Here's how the part is built. I have some questions about the finished solid (model axes, mm). A direction names the side the tool comes from. Give positions to 0.01 mm unless a question says otherwise; leave off trailing zeros. Loops run counter-clockwise (first coordinate to the right, second up) from the corner with the lowest first, then second, coordinate; pieces in that order, holes last. Notation, with made-up numbers: (44, -17.75) - (68, -17.75) arc R7 cw to (68, -7.75) - close; hole circle Ø9 at (56.25, -39.5). An arc over 180 degrees is marked (long way). Use a Markdown table: item, result.
from build123d import *

# Parameters (mm, degrees)
SKETCH2_R           = 4.60375
BOSS_EXTRUDE1_DEPTH = 127
SKETCH3_W           = 76.2
SKETCH3_H           = 31.474420728
CUT_EXTRUDE1_DEPTH  = 254
FILLET1_R           = 2.54
FILLET2_R           = 2.54
FILLET3_R           = 2.54
FILLET4_R           = 2.54
SKETCH4_R           = 1
SKETCH4_W           = 3.81
SKETCH4_H           = 10.16
CUT_EXTRUDE2_DEPTH  = 254


with BuildPart() as part:
    # Sketch2 → Boss-Extrude1 (new body)
    with BuildSketch(Plane.XY):
        with BuildLine():
            Line((-25.661451909, -36.676833639), (-25.661451909, -43.661833639))
            ThreePointArc((-25.661451909, -43.661833639), (-24.917503133, -45.457884863), (-23.121451909, -46.201833639))
            Line((-23.121451909, -46.201833639), (79.748548091, -46.201833639))
            ThreePointArc((79.748548091, -46.201833639), (81.544599316, -45.457884863), (82.288548091, -43.661833639))
            Line((82.288548091, -43.661833639), (82.288548091, -36.676833639))
            ThreePointArc((82.288548091, -36.676833639), (91.813548091, -27.151833639), (101.338548091, -36.676833639))
            Line((101.338548091, -36.676833639), (101.338548091, -46.201833639))
            Line((101.338548091, -46.201833639), (101.338548091, -46.836833639))
            ThreePointArc((101.338548091, -46.836833639), (98.92071457, -52.674000118), (93.083548091, -55.091833639))
            Line((93.083548091, -55.091833639), (-36.456451909, -55.091833639))
            ThreePointArc((-36.456451909, -55.091833639), (-42.293618387, -52.674000118), (-44.711451909, -46.836833639))
            Line((-44.711451909, -46.836833639), (-44.711451909, -46.201833639))
            Line((-44.711451909, -46.201833639), (-44.711451909, -36.676833639))
            ThreePointArc((-44.711451909, -36.676833639), (-35.186451909, -27.151833639), (-25.661451909, -36.676833639))
        make_face()
        with Locations((-35.186451909, -36.676833639)):
            Circle(SKETCH2_R, mode=Mode.SUBTRACT)
        with Locations((91.813548091, -36.676833639)):
            Circle(SKETCH2_R, mode=Mode.SUBTRACT)
    extrude(amount=-BOSS_EXTRUDE1_DEPTH)

    # Sketch3 → Cut-Extrude1 (cut)
    with BuildSketch(Plane(origin=(101.338548091, 0, 0), x_dir=(0, 0, -1), z_dir=(1, 0, 0))):
        with Locations((63.5, -30.464623275)):
            Rectangle(SKETCH3_W, SKETCH3_H)
    extrude(amount=-CUT_EXTRUDE1_DEPTH, mode=Mode.SUBTRACT)

    # Fillet1
    fillet1_edges = [part.edges().sort_by_distance(p)[0] for p in [
        (-33.916451909, -46.201833639, -25.4),
    ]]
    fillet(fillet1_edges, radius=FILLET1_R)

    # Fillet2
    fillet2_edges = [part.edges().sort_by_distance(p)[0] for p in [
        (-33.916451909, -46.201833639, -101.6),
    ]]
    fillet(fillet2_edges, radius=FILLET2_R)

    # Fillet3
    fillet3_edges = [part.edges().sort_by_distance(p)[0] for p in [
        (90.543548091, -46.201833639, -101.6),
    ]]
    fillet(fillet3_edges, radius=FILLET3_R)

    # Fillet4
    fillet4_edges = [part.edges().sort_by_distance(p)[0] for p in [
        (90.543548091, -46.201833639, -25.4),
    ]]
    fillet(fillet4_edges, radius=FILLET4_R)

    # Sketch4 → Cut-Extrude2 (cut)
    with BuildSketch(Plane(origin=(0, -46.201833639, 0), x_dir=(1, 0, 0), z_dir=(0, 1, 0))):
        with Locations(Location((-4.185751909, 106.86, 0), (0, 0, 270))):
            Circle(SKETCH4_R)
        with Locations(Location((60.814248091, 106.86, 0), (0, 0, 270))):
            Circle(SKETCH4_R)
        with Locations(Location((-4.185751909, 22.86, 0), (0, 0, 270))):
            Circle(SKETCH4_R)
        with Locations(Location((60.814248091, 22.86, 0), (0, 0, 270))):
            Circle(SKETCH4_R)
        with Locations((-16.250739794, 64.844309946)):
            Rectangle(SKETCH4_W, SKETCH4_H)
    extrude(amount=-CUT_EXTRUDE2_DEPTH, mode=Mode.SUBTRACT)


solid = part.part
(1) We'd pull the mould along Z, two halves only. Please class faces 1 (the face through (101.339, -42, -20)), 2 (the face through (-35.1, -31.9, -101.6)), 3 (the face through (29, -47, 0)): pulls with the +Z half, pulls with the -Z half, needs draft (parallel to the pull), parting line crosses it, or undercut.
A:
| item | result |
|---|---|
| face 1 | needs draft |
| face 2 | undercut |
| face 3 | pulls with the +Z half |
(2) If I drill on line 1 (X direction, y = -48.5, z = -22.86); line 2 (Y direction, x = 92, z = -6); line 3 (X direction, y = -52.75, z = -106.86), over which ranges is the centre line in solid material (lowest first)?
A:
| item | result |
|---|---|
| line 1 | -44.54 to -5.19, -3.19 to 59.81, 61.81 to 101.17 |
| line 2 | -55.09 to -41.28, -32.08 to -27.15 |
| line 3 | -42.22 to -5.19, -3.19 to 59.81, 61.81 to 98.84 |
(3) Suppose I cut it at A-A on z = -7.5. Count the separate pieces of the cut face and the enclosed holes in it, plus the area to 3 significant figures.
A:
| item | result |
|---|---|
| separate pieces | 1 |
| enclosed holes | 2 |
| area | 1,790 mm2 |
(4) Will this pin go through, and if not, where does the flat tip stop? pin 1 (10 mm diameter, centred on x = 60, z = -81, fed in from +Y).
A:
| item | result |
|---|---|
| pin 1 | y = -46.2 |
(5) Suppose I cut it at B-B on y = -50.75. Write out the boundary of the cut face in (x, z).
A:
| item | result |
|---|---|
| outline | (-43.73, -127) - (100.35, -127) - (100.35, 0) - (-43.73, 0) - close; hole (-18.16, -69.92) - (-14.35, -69.92) - (-14.35, -59.76) - (-18.16, -59.76) - close; hole circle Ø2 at (-4.19, -106.86); hole circle Ø2 at (-4.19, -22.86); hole circle Ø2 at (60.81, -106.86); hole circle Ø2 at (60.81, -22.86) |
(6) Suppose I cut it at C-C on z = -89. Write out the boundary of the cut face in (x, y) (3 decimals), plus the area to 3 significant figures.
A:
| item | result |
|---|---|
| outline | (-44.711, -46.837) arc R8.255 ccw to (-36.456, -55.092) - (93.084, -55.092) arc R8.255 ccw to (101.339, -46.837) - (101.339, -46.202) - (-44.711, -46.202) - close |
| area | 1,270 mm2 |
(7) On a 3-axis mill with a long thin cutter (end or side, diameter ignored), from which of +Z, -Z, +X, -X, +Y, -Y can I reach the whole of each face in a straight line? I mean faces 4 (the face through (-25.661, -40, -13)), 5 (the face through (-14.346, -51, -65)), 6 (the face through (-38.84, -39.48, -114.12)), 7 (the face through (91.9, -31.9, -25.4)). Say none if no direction works.
A:
| item | result |
|---|---|
| face 4 | +Z, -Z, +Y |
| face 5 | +Y, -Y |
| face 6 | +Z, -Z |
| face 7 | +X, -X, +Y |
(8) Suppose I cut it at D-D on y = -29.5. Write out the boundary of the cut face in (x, z).
A:
| item | result |
|---|---|
| outline | (-41.45, -127) - (-28.92, -127) - (-28.92, -101.6) - (-41.45, -101.6) - close; (-41.45, -25.4) - (-28.92, -25.4) - (-28.92, 0) - (-41.45, 0) - close; (85.55, -127) - (98.08, -127) - (98.08, -101.6) - (85.55, -101.6) - close; (85.55, -25.4) - (98.08, -25.4) - (98.08, 0) - (85.55, 0) - close |
